Autodesk Inventor part; units mm, degrees
ref_plane "Work Plane1" through (82.55, 89.535, -212.09) normal (0, 0, 1) x (1, 0, 0)
ref_plane "YZ Plane" through (0, 0, 0) normal (1, 0, 0) x (0, 1, 0)
ref_plane "XZ Plane" through (0, 0, 0) normal (0, 1, 0) x (-1, 0, 0)
sketch "Sketch1" plane through (0, 0, 0) normal (1, 0, 0) x (0, 1, 0)
  line L0 (0, 0) -> (228.6, 0)
  line L1 (228.6, 0) -> (228.6, -424.18)
  line L2 (228.6, -424.18) -> (0, -424.18)
  line L3 (0, -424.18) -> (0, 0)
  point P0 (0, 0)
  dimension "d0" = 424.18
  dimension "d1" = 228.6
extrude "Extrusion1" add sketch "Sketch1" along normal blind 165.1
sketch "Sketch2" plane through (165.1, 0, 0) normal (1, 0, 0) x (0, 0, -1)
  line L0 (0, 0) -> (424.18, 0) construction
  line L1 (12.7, 0) -> (411.48, 0)
  line L2 (411.48, 0) -> (411.48, 165.1)
  line L3 (411.48, 165.1) -> (12.7, 165.1)
  line L4 (12.7, 165.1) -> (12.7, 0)
  line L5 (0, 228.6) -> (0, 0) construction
  line L6 (424.18, 0) -> (424.18, 228.6) construction
  dimension "d4" = 398.78
  dimension "d5" = 165.1
  dimension "d6" = 12.7
  dimension "d7" = 12.7
extrude "Extrusion2" cut sketch "Sketch2" against normal blind 148.59
sketch "Sketch3" plane through (0, 0, 0) normal (0, 0, 1) x (1, 0, 0)
  line L0 (165.1, 228.6) -> (165.1, 0)
  line L1 (165.1, 89.535) -> (82.55, 89.535)
  line L2 (69.215, 89.535) -> (69.215, 62.865) construction
  line L3 (82.55, 62.865) -> (165.1, 62.865)
  line L4 (165.1, 62.865) -> (165.1, 89.535)
  line L5 (0, 0) -> (165.1, 0)
  arc A0 (82.55, 89.535) -> (82.55, 62.865) centre (82.55, 76.2) ccw
  dimension "d10" = 95.885
  dimension "d11" = 26.67
  dimension "d12" = 62.865
extrude "Extrusion3" cut sketch "Sketch3" against normal blind 457.2
sketch "Sketch4" plane through (0, 228.6, 0) normal (0, 1, 0) x (1, 0, 0)
  line L0 (165.1, 12.7) -> (165.1, 411.48) construction
  line L1 (165.1, 12.7) -> (16.51, 12.7) construction
  line L2 (16.51, 12.7) -> (16.51, 411.48) construction
  line L3 (165.1, 411.48) -> (16.51, 411.48) construction
  line L4 (0, 424.18) -> (165.1, 424.18) construction
  line L5 (0, 424.18) -> (165.1, 424.18) construction
  circle A0 centre (82.55, 353.06) radius 43.815
  line L6 (0, 0) -> (0, 424.18) construction
  circle A1 centre (82.55, 259.08) radius 43.815
  line L7 (0, 212.09) -> (165.1, 212.09) construction
  line L8 (165.1, 424.18) -> (165.1, 0) construction
  circle A2 centre (82.55, 71.12) radius 43.815
  circle A3 centre (82.55, 165.1) radius 43.815
  dimension "d15" = 87.63
  dimension "d16" = 82.55
  dimension "d17" = 58.42
  dimension "d18" = 87.63
  dimension "d19" = 93.98
  dimension "d20" = 82.55
extrude "Extrusion4" cut sketch "Sketch4" against normal blind 76.2
sketch "Sketch5" plane through (0, 228.6, 0) normal (0, 1, 0) x (1, 0, 0)
  circle A0 centre (82.55, 165.1) radius 43.815
  circle A1 centre (82.55, 353.06) radius 43.815
  circle A2 centre (82.55, 259.08) radius 43.815
  circle A3 centre (82.55, 71.12) radius 43.815
  line L0 (0, 0) -> (0, 424.18)
  line L1 (0, 0) -> (165.1, 0)
  line L2 (165.1, 424.18) -> (165.1, 0)
  line L3 (0, 424.18) -> (165.1, 424.18)
  point P0 (0, 0)
extrude "Extrusion5" add sketch "Sketch5" along normal blind 53.34
sketch "Sketch7" plane through (0, 0, 0) normal (-1, 0, 0) x (0, 0, 1)
  line L0 (0, 0) -> (0, 281.94)
  line L1 (-424.18, 281.94) -> (0, 281.94)
  line L2 (-424.18, 281.94) -> (-424.18, 0)
  line L3 (-424.18, 0) -> (0, 0)
  point P0 (0, 0)
extrude "Extrusion6" add sketch "Sketch7" along normal blind 19.05
sketch "Sketch8" plane through (16.51, 0, 0) normal (1, 0, 0) x (0, 0, -1)
  line L0 (411.48, 0) -> (12.7, 0)
  line L1 (411.48, 165.1) -> (411.48, 0)
  line L2 (12.7, 165.1) -> (411.48, 165.1)
  line L3 (12.7, 0) -> (12.7, 165.1)
  point P0 (0, 0)
extrude "Extrusion7" cut sketch "Sketch8" against normal blind 19.05
sketch "Sketch12" plane through (165.1, 0, 0) normal (1, 0, 0) x (0, 0, -1)
  line L0 (0, 89.535) -> (12.7, 89.535) construction
  line L1 (3.302, 89.535) -> (9.398, 89.535)
  line L2 (9.398, 89.535) -> (9.398, 92.583)
  line L3 (9.398, 92.583) -> (3.302, 92.583)
  line L4 (3.302, 92.583) -> (3.302, 89.535)
  line L5 (0, 89.535) -> (0, 281.94) construction
  line L6 (12.7, 89.535) -> (12.7, 62.865) construction
  line L7 (0, 89.535) -> (12.7, 89.535) construction
  line L8 (0, 62.865) -> (0, 89.535) construction
  line L9 (0, 62.865) -> (12.7, 62.865) construction
  line L10 (0, 62.865) -> (0, 89.535) construction
  line L11 (0, 76.2) -> (12.7, 76.2) construction
  line L12 (3.302, 62.865) -> (9.398, 62.865)
  line L13 (9.398, 62.865) -> (9.398, 59.817)
  line L14 (9.398, 59.817) -> (3.302, 59.817)
  line L15 (3.302, 59.817) -> (3.302, 62.865)
  point P0 (0, 0)
  dimension "d44" = 6.096
  dimension "d45" = 3.048
  dimension "d46" = 3.302
extrude "Extrusion11" cut sketch "Sketch12" against normal blind 82.55
sketch "Sketch13" plane through (-19.05, 0, 0) normal (0, -1, 0) x (1, 0, 0)
  line L0 (16.51, -12.7) -> (184.15, -12.7)
  line L1 (184.15, 0) -> (184.15, -12.7)
  line L2 (0, 0) -> (184.15, 0)
  line L3 (0, -424.18) -> (0, 0)
  line L4 (184.15, -424.18) -> (0, -424.18)
  line L5 (184.15, -411.48) -> (184.15, -424.18)
  line L6 (184.15, -411.48) -> (16.51, -411.48)
  line L7 (16.51, -411.48) -> (16.51, -12.7)
  point P0 (19.05, 0)
extrude "Extrusion12" add sketch "Sketch13" along normal blind 5.08
ref_plane "Work Plane1" through (82.55, 89.535, -212.09) normal (0, 0, 1) x (1, 0, 0)
mirror "Mirror1" about plane through (82.55, 89.535, -212.09) normal (0, 0, 1) of "Extrusion11"
sketch "Sketch15" plane through (165.1, 0, 0) normal (1, 0, 0) x (0, 0, -1)
  line L0 (3.302, 59.817) -> (8.89, 59.817)
  line L1 (8.89, 59.817) -> (8.89, 57.912)
  line L2 (8.89, 57.912) -> (3.302, 57.912)
  line L3 (3.302, 57.912) -> (3.302, 59.817)
  line L4 (9.398, 59.817) -> (3.302, 59.817)
  point P0 (0, 0)
  dimension "d55" = 5.588
  dimension "d56" = 1.905
extrude "Extrusion14" add sketch "Sketch15" along normal blind 3.81
sketch "Sketch17" plane through (165.1, 57.912, -3.302) normal (0, 0, 1) x (1, 0, 0)
  line L0 (0, 1.905) -> (3.81, 1.905)
  line L1 (3.81, 1.905) -> (0, 1.905)
  line L2 (0, 1.905) -> (0, 0.889)
  line L3 (0, 0.889) -> (3.81, 0.889)
  line L4 (3.81, 0.889) -> (3.81, 1.905)
  point P0 (-165.1, -57.912)
  dimension "d60" = 3.81
  dimension "d61" = 1.016
extrude "Extrusion15" cut sketch "Sketch17" against normal blind 25.4
sketch "Sketch18" plane through (165.1, 57.912, -3.302) normal (0, 0, 1) x (1, 0, 0)
  line L0 (0, 1.905) -> (-82.55, 1.905) construction
  line L1 (3.81, 0) -> (3.81, 0.889)
  line L2 (1.905, 2.9464) -> (3.81, 0.889)
  line L3 (3.81, 0.889) -> (1.905, 0.889)
  line L4 (1.905, 0.889) -> (1.905, 2.9464)
  line L5 (0, 4.953) -> (0, -62.992)
  point P0 (-165.1, -57.912)
  dimension "d64" = 1.905
  dimension "d65" = 2.0574
extrude "Extrusion16" add sketch "Sketch18" against normal blind 5.588
sketch "Sketch19" plane through (165.1, 57.912, -8.89) normal (0, -1, 0) x (1, 0, 0)
  line L0 (0, 0) -> (0, 5.588)
  line L1 (0, 0) -> (3.81, 0)
  line L2 (3.81, 5.588) -> (3.81, 0)
  line L3 (0, 5.588) -> (3.81, 5.588)
  point P0 (-165.1, 8.89)
extrude "Extrusion17" add sketch "Sketch19" along normal blind 1.524
mirror "Mirror2" about plane through (82.55, 89.535, -212.09) normal (0, 0, 1) of "Extrusion14", "Extrusion15", "Extrusion16", "Extrusion17"
sketch "Sketch21" plane through (82.55, 89.535, 0) normal (0, 0, 1) x (1, 0, 0)
  line L0 (49.9587, -43.0228) -> (93.9109, -43.0228)
  line L1 (93.9109, -43.0228) -> (93.9109, 15.0648)
  line L2 (93.9109, 15.0648) -> (49.9587, 15.0648)
  line L3 (49.9587, 15.0648) -> (49.9587, -43.0228)
  point P0 (-82.55, -89.535)
extrude "Extrusion18" cut sketch "Sketch21" against normal blind 25.4 keep common part
sketch "Sketch22" plane through (132.5087, 104.5998, 0) normal (0, 0, 1) x (1, 0, 0)
  line L0 (0, -58.0876) -> (32.5913, -58.0876)
  line L1 (0, 0) -> (16.2957, 0)
  line L2 (16.2957, 0) -> (16.2957, -58.0876)
  line L3 (16.2957, -58.0876) -> (0, -58.0876)
  line L4 (0, -58.0876) -> (0, 0)
  point P0 (-132.5087, -104.5998)
extrude "Extrusion19" add sketch "Sketch22" along normal blind 6.35
sketch "Sketch23" plane through (148.8043, 62.865, 0) normal (1, 0, 0) x (0, 0, -1)
  line L0 (0, 26.67) -> (0, 41.7348)
  line L1 (0, 29.21) -> (-1.27, 29.21)
  line L2 (-1.27, 29.21) -> (-1.27, -2.54)
  line L3 (-1.27, -2.54) -> (0, -2.54)
  line L4 (0, -2.54) -> (0, 29.21)
  line L5 (0, 26.67) -> (3.302, 26.67)
  line L6 (3.302, 0) -> (0, 0)
  point P0 (0, -62.865)
  dimension "d74" = 1.27
  dimension "d75" = 2.54
  dimension "d76" = 2.54
extrude "Extrusion20" cut sketch "Sketch23" against normal blind 25.4
sketch "Sketch9" plane through (0, 281.94, 0) normal (0, 1, 0) x (1, 0, 0)
  line L0 (146.05, 19.05) -> (146.05, 405.13)
  line L1 (0, 405.13) -> (0, 19.05)
  line L2 (165.1, 424.18) -> (-19.05, 424.18) construction
  line L3 (-19.05, 0) -> (-19.05, 424.18) construction
  line L4 (165.1, 0) -> (165.1, 424.18) construction
  line L5 (165.1, 0) -> (-19.05, 0) construction
  circle A0 centre (82.55, 71.12) radius 43.815 construction
  circle A1 centre (82.55, 259.08) radius 43.815 construction
  circle A2 centre (82.55, 353.06) radius 43.815 construction
  circle A3 centre (82.55, 165.1) radius 43.815 construction
  line L6 (165.1, 0) -> (-19.05, 0) construction
  line L7 (165.1, 0) -> (165.1, 424.18) construction
  line L8 (165.1, 424.18) -> (-19.05, 424.18) construction
  line L9 (-19.05, 0) -> (-19.05, 424.18) construction
  line L10 (146.05, 405.13) -> (117.7739, 405.13)
  line L11 (47.3261, 405.13) -> (0, 405.13)
  arc A4 (47.3261, 405.13) -> (40.7894, 306.07) centre (82.55, 353.06) ccw
  arc A5 (124.3106, 306.07) -> (117.7739, 405.13) centre (82.55, 353.06) ccw
  arc A6 (40.7894, 306.07) -> (40.7894, 212.09) centre (82.55, 259.08) ccw
  arc A7 (124.3106, 212.09) -> (107.2668, 316.8822) centre (82.55, 259.08) ccw
  arc A8 (40.7894, 212.09) -> (40.7894, 118.11) centre (82.55, 165.1) ccw
  arc A9 (124.3106, 118.11) -> (124.3106, 212.09) centre (82.55, 165.1) ccw
  line L12 (0, 19.05) -> (47.3261, 19.05)
  line L13 (117.7739, 19.05) -> (146.05, 19.05)
  arc A10 (40.7894, 118.11) -> (47.3261, 19.05) centre (82.55, 71.12) ccw
  arc A11 (117.7739, 19.05) -> (124.3106, 118.11) centre (82.55, 71.12) ccw
  point P0 (0, 0)
  dimension "d30" = 19.05
  dimension "d31" = 19.05
sketch "Sketch10" plane through (0, 281.94, -19.05) normal (1, 0, 0) x (0, 0, -1)
  line L0 (405.13, 0) -> (405.13, -281.94)
  line L1 (-19.05, 0) -> (405.13, 0)
  line L2 (405.13, -101.6) -> (-19.05, -101.6)
  line L3 (-19.05, -101.6) -> (-19.05, 0)
  line L4 (-19.05, 0) -> (405.13, 0)
  line L5 (405.13, 0) -> (405.13, -101.6)
  line L6 (0, 0) -> (386.08, 0)
  line L7 (0, 0) -> (0, -101.6)
  line L8 (0, -101.6) -> (386.08, -101.6)
  line L9 (386.08, 0) -> (386.08, -101.6)
  point P0 (-19.05, -281.94)
  dimension "d39" = 0
sketch "Sketch11" plane through (0, 281.94, 0) normal (0, 1, 0) x (1, 0, 0)
  circle A0 centre (82.55, 71.12) radius 43.815 construction
  line L0 (19.05, 19.05) -> (19.05, 0)
  line L1 (19.05, 0) -> (47.3261, 0)
  line L2 (47.3261, 0) -> (47.3261, 19.05)
  line L3 (47.3261, 19.05) -> (19.05, 19.05)
  line L4 (19.05, 19.05) -> (19.05, 0)
  line L5 (165.1, 424.18) -> (19.05, 424.18)
  line L6 (47.3261, 405.13) -> (19.05, 405.13)
  line L7 (19.05, 405.13) -> (19.05, 424.18)
  line L8 (19.05, 424.18) -> (47.3261, 424.18)
  line L9 (47.3261, 424.18) -> (47.3261, 405.13)
  point P0 (0, 0)
properties part number "EngineClipTestBlock"
Geometry check sheet. Reference: the model listing, model coordinates, mm. A direction names the side the tool comes from. Coordinates: 2 decimals unless noted, no trailing zeros. Order: outer loops, then holes, each group sorted by start corner. A loop starts at its lowest first (then second) coordinate and runs counter-clockwise, first axis right, second up.
Item 1: Section check D-D (z = -7.25). Enter the section's corners in (x, y) (3 decimals).
Item 2: Tool access check on faces 1 (the flat face through (165.1, 97, -6)), 2 (the flat face through (149, 89.535, -2)), 3 (the flat face through (149, 91, -9.398)), 4 (the flat face through (167, 56.388, -6)). Record the directions out of +Z, -Z, +X, -X, +Y, -Y that give a thin tool (end or side, any length) a straight path to the whole face; none if there is none.
Item 3: Section check A-A (z = -1). Enter the section's corners in (x, y) (3 decimals), plus the area to 3 significant figures.
Item 4: Section check B-B (x = 153). Enter the section's corners in (y, z) (3 decimals), plus the area to 3 significant figures.
Item 5: Section check C-C (y = 58). Enter the section's corners in (x, z), plus the area to 3 significant figures.
Item 6: Depth check by flat-ended pin: pin 1 (1.1 mm diameter, centred on x = 166.5, z = -5.5, fed in from -Y); pin 2 (18 mm diameter, centred on x = 137.5, y = 79, fed in from -Z); pin 3 (6.5 mm diameter, centred on y = 97, z = -4.5, fed in from +X); pin 4 (4 mm diameter, centred on y = 66.5, z = -2, fed in from -X). Enter the tip coordinate at first touch or a pass-through.
Item 7: Scan lines: line 1 along Y through (x, z) = (156, -7.75); line 2 along Y through (x, z) = (163.5, -11) (3 decimals); line 3 along Z through (x, y) = (150, 51.5). Record each from-to range of solid material in increasing order.
Item 8: Mould release check, pull along Z, two halves, no side actions. Record for faces 5 (the flat face through (149, 104.6, -5)), 6 (the flat face through (149, 61, -3.302)), 7 (the flat face through (141, 76, 6.35)): released by +Z, released by -Z, zero draft, split by the parting line, or undercut.
Check sheet entries:
1. outline: (132.509, 46.512) - (165.1, 46.512) - (165.1, 56.388) - (168.91, 56.388) - (168.91, 58.801) - (167.005, 60.858) - (167.005, 58.801) - (165.1, 58.801) - (165.1, 59.817) - (132.509, 59.817) - close; (132.509, 92.583) - (165.1, 92.583) - (165.1, 104.6) - (132.509, 104.6) - close
2. face 1: +Z, -Z, +X, +Y
2. face 2: -Z, +X, -X
2. face 3: +X, -X
2. face 4: +Z, -Z, +X, -Y
3. outline: (132.509, 46.512) - (165.1, 46.512) - (165.1, 62.865) - (132.509, 62.865) - close; (132.509, 89.535) - (165.1, 89.535) - (165.1, 104.6) - (132.509, 104.6) - close
3. area: 1,020 mm2
4. outline: (46.512, -12.7) - (62.865, -12.7) - (62.865, -9.398) - (59.817, -9.398) - (59.817, -3.302) - (62.865, -3.302) - (62.865, 0) - (46.512, 0) - close; (89.535, -12.7) - (104.6, -12.7) - (104.6, 0) - (89.535, 0) - (89.535, -3.302) - (92.583, -3.302) - (92.583, -9.398) - (89.535, -9.398) - close
4. area: 362 mm2
5. outline: (132.51, -12.7) - (165.1, -12.7) - (165.1, -8.89) - (168.91, -8.89) - (168.91, -3.3) - (165.1, -3.3) - (165.1, 0) - (148.8, 0) - (148.8, 6.35) - (132.51, 6.35) - close
5. area: 539 mm2
6. pin 1: stops at y = 56.39
6. pin 2: stops at z = 1.27
6. pin 3: stops at x = 165.1
6. pin 4: passes through
7. line 1: y = 46.51 to 59.82, 92.58 to 104.6
7. line 2: y = 46.512 to 62.865, 89.535 to 104.6
7. line 3: z = -12.7 to 0
8. face 5: zero draft
8. face 6: undercut
8. face 7: released by +Z
